from build123d import *

# Parameters (mm, degrees)
F0_R     = 3.05
F1_DEPTH = 3.9
F2_R     = 3.05
F2_R_2   = 1.4
F3_DEPTH = 1


with BuildPart() as f1:
    # F0 (on Front) → F1 (new body)
    with BuildSketch(Plane.XZ):
        with BuildLine():
            ThreePointArc((7.5383832306, 6.5705995365), (8.2516737727, 5.6488830709), (8.8528781464, 4.6504353048))
            ThreePointArc((8.8528781464, 4.6504353048), (8.9284772277, 4.6763186551), (9.0050498972, 4.6991614919))
            ThreePointArc((9.0050498972, 4.6991614919), (12.9883654229, 10.7400635802), (7.5383832306, 15.5))
            Line((7.5383832306, 15.5), (-7.4616167694, 15.5))
            ThreePointArc((-7.4616167694, 15.5), (-12.9115989618, 10.7400635802), (-8.9282834361, 4.6991614919))
            ThreePointArc((-8.9282834361, 4.6991614919), (-8.8845194647, 4.6865143215), (-8.8410548965, 4.6728736679))
            ThreePointArc((-8.8410548965, 4.6728736679), (-8.2115228808, 5.7070913763), (-7.4616167694, 6.6576478719))
            ThreePointArc((-7.4616167694, 6.6576478719), (-4.0880020353, 9.1262390589), (0, 10))
            ThreePointArc((0, 10), (4.1408939032, 9.1023622034), (7.5383832306, 6.5705995365))
        make_face()
        with BuildLine():
            ThreePointArc((-7.4616167694, 6.6576478719), (-8.2115228808, 5.7070913763), (-8.8410548965, 4.6728736679))
            ThreePointArc((-8.8410548965, 4.6728736679), (-7.84280181, 3.9460786917), (-7.4616167694, 2.7715838526))
            Line((-7.4616167694, 2.7715838526), (-7.4616167694, 6.6576478719))
        make_face()
        with BuildLine():
            ThreePointArc((-8.8410548965, 4.6728736679), (-2.4072236118, -9.7059401648), (10, 0))
            ThreePointArc((10, 0), (9.7089850516, 2.3949132068), (8.8528781464, 4.6504353048))
            ThreePointArc((8.8528781464, 4.6504353048), (7.8996321561, 3.9180980984), (7.5383832306, 2.7715838526))
            Line((7.5383832306, 2.7715838526), (7.5383832306, 6.5705995365))
            ThreePointArc((7.5383832306, 6.5705995365), (4.1408939032, 9.1023622034), (0, 10))
            ThreePointArc((0, 10), (-4.0880020353, 9.1262390589), (-7.4616167694, 6.6576478719))
            Line((-7.4616167694, 6.6576478719), (-7.4616167694, 2.7715838526))
            ThreePointArc((-7.4616167694, 2.7715838526), (-7.84280181, 3.9460786917), (-8.8410548965, 4.6728736679))
        make_face()
        Circle(F0_R, mode=Mode.SUBTRACT)
        with BuildLine():
            ThreePointArc((7.5383832306, 2.7715838526), (7.8996321561, 3.9180980984), (8.8528781464, 4.6504353048))
            ThreePointArc((8.8528781464, 4.6504353048), (8.2516737727, 5.6488830709), (7.5383832306, 6.5705995365))
            Line((7.5383832306, 6.5705995365), (7.5383832306, 2.7715838526))
        make_face()
    extrude(amount=F1_DEPTH)

    # F2 (on face) → F3 (join)
    with BuildSketch(Plane.XZ.offset(3.9)):
        with BuildLine():
            ThreePointArc((-8.9282834361, 4.6991614919), (-8.8845194647, 4.6865143215), (-8.8410548965, 4.6728736679))
            ThreePointArc((-8.8410548965, 4.6728736679), (-0.0126813778, -9.9999919591), (8.8528781464, 4.6504353048))
            ThreePointArc((8.8528781464, 4.6504353048), (8.9284772277, 4.6763186551), (9.0050498972, 4.6991614919))
            ThreePointArc((9.0050498972, 4.6991614919), (12.9883654229, 10.7400635802), (7.5383832306, 15.5))
            Line((7.5383832306, 15.5), (-7.4616167694, 15.5))
            ThreePointArc((-7.4616167694, 15.5), (-12.9115989618, 10.7400635802), (-8.9282834361, 4.6991614919))
        make_face()
        Circle(F2_R, mode=Mode.SUBTRACT)
        Circle(F2_R)
        Circle(F2_R_2, mode=Mode.SUBTRACT)
    extrude(amount=F3_DEPTH)

    # F5 (on offset) → F6 (revolve)
    with BuildSketch(Plane.XY.offset(10)):
        with BuildLine():
            Line((-7.5, -5.7002530202), (-7.5, -10.7002530202))
            ThreePointArc((-7.5, -10.7002530202), (-5.2926553092, -9.3739776115), (-5.427348204, -6.8023565532))
            ThreePointArc((-5.427348204, -6.8023565532), (-6.3262754087, -5.9929083295), (-7.5, -5.7002530202))
        make_face()
        with BuildLine():
            ThreePointArc((-7.5, -5.7002530202), (-6.3262754087, -5.9929083295), (-5.427348204, -6.8023565532))
            Line((-5.427348204, -6.8023565532), (-5.427348204, -4.8014420412))
            Line((-5.427348204, -4.8014420412), (-7.5, -4.8014420412))
            Line((-7.5, -4.8014420412), (-7.5, -4.8982134417))
            Line((-7.5, -4.8982134417), (-7.5, -5.7002530202))
        make_face()
    revolve(axis=Axis((-7.5, -4.8982134417, 10), (0, -1, 0)))

    # F5 (on offset) → F7 (revolve)
    with BuildSketch(Plane.XY.offset(10)):
        with BuildLine():
            ThreePointArc((7.5, -5.7002530202), (8.6737245913, -5.9929083295), (9.572651796, -6.8023565532))
            Line((9.572651796, -6.8023565532), (9.572651796, -4.7845813774))
            Line((9.572651796, -4.7845813774), (7.5, -4.7845813774))
            Line((7.5, -4.7845813774), (7.5, -5.7002530202))
        make_face()
        with BuildLine():
            Line((7.5, -5.7002530202), (7.5, -10.7002530202))
            ThreePointArc((7.5, -10.7002530202), (9.7073446908, -9.3739776115), (9.572651796, -6.8023565532))
            ThreePointArc((9.572651796, -6.8023565532), (8.6737245913, -5.9929083295), (7.5, -5.7002530202))
        make_face()
    revolve(axis=Axis((7.5, -4.7317600206, 10), (0, -1, 0)))


solid = f1.part
Here's how the part is built. I have some questions about the finished solid (model axes, mm). A direction names the side the tool comes from. Give positions to 0.01 mm unless a question says otherwise; leave off trailing zeros. Write each loop counter-clockwise with the first axis right and the second up, starting at its lowest first coordinate (ties: lowest second). Pieces come first, ordered by that corner, then holes. Notation, with made-up numbers: (46, -37.5) -> (91, -37.5) arc R24 ccw to (91, -7.5) -> close; hole circle Ø11 at (31.5, 80). An arc over 180 degrees is marked (long way). Use one line per item in the form item = value. Start each with the question number.
1. Imagine slicing it at A-A on y = -4.5. List the corners of the cut face in (x, z) for me, plus the area to 3 significant figures.
2. Thinking about a two-plate mould opening in Z: for faces 4 (the face through (0, 0, 6)), 5 (the face through (-9.145, -5.838, 8.739)), 6 (the face through (-1.4, -4.39, 0.06)), which applies, +Z half, -Z half, draft (parallel to the pull), parting line (faces both ways), or undercut?
3. On a 3-axis mill with a long thin cutter (end or side, diameter ignored), from which of +Z, -Z, +X, -X, +Y, -Y can I reach the whole of each face in a straight line? I mean faces 1 (the face through (7.051, -5.838, 7.977)), 2 (the face through (-12.896, -2.416, 10.849)), 3 (the face through (-3.047, -1.923, 0.134)). Say none if no direction works.
4. Imagine slicing it at D-D on y = -2.75. List the corners of the cut face in (x, z) for me.
5. Imagine slicing it at C-C on y = -6. List the corners of the cut face in (x, z) for me.
6. Will these pins go through, and if not, where does the flat tip stop? pin 1 Ø6 at (y, z) = (-5, -3.5) entering from -X; pin 2 Ø1.5 at (y, z) = (-7.5, 9.5) entering from +X; pin 3 Ø7.5 at (x, z) = (4, 0) entering from -Y.
7. If I drill on L1, parallel to Z at x = 0, y = -1.75; L2, parallel to Z at x = 0, y = -4.5; L3, parallel to Y at x = -9.5, z = 5.5, over which ranges is the centre line in solid material (lowest first)?
8. Imagine slicing it at B-B on x = 0. List the corners of the cut face in (y, z) for me.
Entries:
q1.outline = (-8.93, 4.7) arc R2 cw to (-8.84, 4.67) arc R10 ccw (long way) to (8.85, 4.65) arc R2 cw to (9.01, 4.7) arc R5.5 ccw to (7.54, 15.5) -> (-7.46, 15.5) arc R5.5 ccw to start; hole circle Ø2.8 at (0, 0)
q1.area = 498 mm²
q2.face_4 = draft
q2.face_5 = parting line
q2.face_6 = undercut
q3.face_1 = none
q3.face_2 = -X, +Y, -Y
q3.face_3 = +Y
q4.outline = (-8.93, 4.7) arc R2 cw to (-8.84, 4.67) arc R10 ccw (long way) to (8.85, 4.65) arc R2 cw to (9.01, 4.7) arc R5.5 ccw to (7.54, 15.5) -> (-7.46, 15.5) arc R5.5 ccw to start; hole circle Ø6.1 at (0, 0)
q5.outline = circle Ø4.15 at (-7.5, 10); circle Ø4.15 at (7.5, 10)
q6.pin_1 = -9.99
q6.pin_2 = 10
q6.pin_3 = -4.9
q7.L1 = -10 to -3.05, 3.05 to 15.5
q7.L2 = -10 to -1.4, 1.4 to 15.5
q7.L3 = -4.9 to 0
q8.outline = (-4.9, -10) -> (0, -10) -> (0, -3.05) -> (-3.9, -3.05) -> (-3.9, -1.4) -> (-4.9, -1.4) -> close; (-4.9, 1.4) -> (-3.9, 1.4) -> (-3.9, 3.05) -> (0, 3.05) -> (0, 15.5) -> (-4.9, 15.5) -> close
